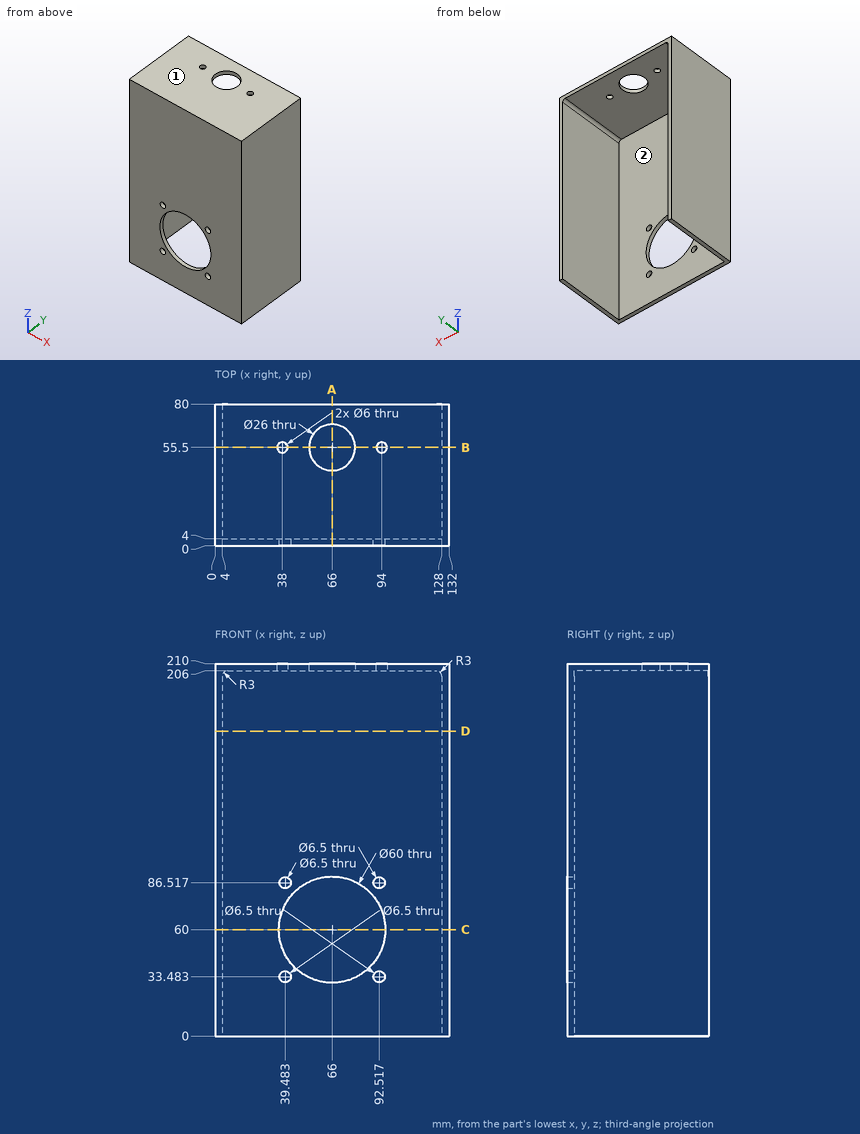
Could you check a few things on this drawing? It's one solid part, dimensions in mm from its lowest x, y, z. A direction names the side the tool comes from. Coordinates: 2 decimals unless noted, no trailing zeros. Loops run counter-clockwise (first coordinate to the right, second up) from the corner with the lowest first, then second, coordinate; pieces in that order, holes last. Notation, with made-up numbers: (5, -8) - (38, -8) arc R23 ccw to (38, 9) - close; hole circle Ø4 at (7.25, -35). An arc over 180 degrees is marked (long way). Return JSON: item names as keys, results as strings. Group by question number.
Item 1: I need wall thicknesses on line 1 (X direction, y = 55, z = 207); line 2 (X direction, y = 2.6, z = 60); line 3 (X direction, y = 46.5, z = 156). Which ranges of each line are inside material? Lowest first, please. Write a range as from..to.
Item 2: On a 3-axis mill with a long thin cutter (end or side, diameter ignored), from which of +Z, -Z, +X, -X, +Y, -Y can I reach the whole of each face in a straight line? I mean the marked faces 1 and 2. Say none if no direction works.
Item 3: Will this pin go through, and if not, where does the flat tip stop? P1, Ø8, axis at x = 37, y = 66.5, coming from the -Z side.
Item 4: If we section it at B-B on y = 55.5: Write out the boundary of the cut face in (x, z), and give its area (3 significant figures).
Item 5: If we section it at A-A on x = 66: Write out the boundary of the cut face in (y, z), and give its area (3 significant figures).
Item 6: If we section it at D-D on z = 172: Write out the boundary of the cut face in (x, y).
Item 7: If we section it at C-C on z = 60: Write out the boundary of the cut face in (x, y).
Calculated:
{
 "1": {"line 1": "x = 0..35.04, 40.96..53.01, 78.99..91.04, 96.96..132", "line 2": "x = 0..36, 96..132", "line 3": "x = 0..4, 128..132"},
 "2": {"face 1": "+Z, +X, -X, +Y, -Y", "face 2": "-Z, +Y"},
 "3": {"P1": "stops at z = 206"},
 "4": {"outline": "(0, 0) - (4, 0) - (4, 203) arc R3 cw to (7, 206) - (35, 206) - (35, 210) - (0, 210) - close; (41, 206) - (53, 206) - (53, 210) - (41, 210) - close; (79, 206) - (91, 206) - (91, 210) - (79, 210) - close; (97, 206) - (125, 206) arc R3 cw to (128, 203) - (128, 0) - (132, 0) - (132, 210) - (97, 210) - close", "area": "2,030 mm^2"},
 "5": {"outline": "(0, 0) - (4, 0) - (4, 30) - (0, 30) - close; (0, 90) - (4, 90) - (4, 206) - (42.5, 206) - (42.5, 210) - (0, 210) - close; (68.5, 206) - (80, 206) - (80, 210) - (68.5, 210) - close", "area": "800 mm^2"},
 "6": {"outline": "(0, 0) - (132, 0) - (132, 80) - (128, 80) - (128, 4) - (4, 4) - (4, 80) - (0, 80) - close"},
 "7": {"outline": "(0, 0) - (36, 0) - (36, 4) - (4, 4) - (4, 80) - (0, 80) - close; (96, 0) - (132, 0) - (132, 80) - (128, 80) - (128, 4) - (96, 4) - close"}
}
